Geometry: final body of the model. Coordinates: model frame, mm. A direction names the side the tool comes from. Give positions to 0.01 mm unless a question says otherwise; leave off trailing zeros. Write each loop counter-clockwise with the first axis right and the second up, starting at its lowest first coordinate (ties: lowest second). Pieces come first, ordered by that corner, then holes.
Q1. Reachability of faces 1 (the face through (2, 0, -5)), 2 (the face through (0, 25.4, 0)) from +Z, -Z, +X, -X, +Y, -Y: full face, straight path, thin tool, end or side. Return the list, or none.
Q2. Cut plane B-B on y = 4.5. Return the cut outline in (x, z), plus the area to 3 significant figures.
Q3. Cut plane C-C on x = 2.75. Return the cut outline in (y, z).
Q4. Pin query (flat end, axial travel): pin 1 (1.5 mm diameter, centred on y = 12, z = -2.5, fed in from +X); pin 2 (4 mm diameter, centred on x = -5, y = 16, fed in from +Z); pin 3 (4 mm diameter, centred on x = 1.5, y = 3.5, fed in from -Z); pin 4 (1.7 mm diameter, centred on x = -4.5, z = 5.5, fed in from -Y). Return the tip coordinate at first contact, or that it passes through.
Q5. Cut plane D-D on x = 4.25. Return the cut outline in (y, z), plus the area to 3 significant figures.
Q6. Cut plane A-A on x = 0. Return the cut outline in (y, z).
Q7. Line query: L1, parallel to X at y = 8.5, z = 0; L2, parallel to Z at x = 0.25, y = 1.25; L3, parallel to Y at x = -5, z = 2.25. Output: solid intervals per line, ascending.
```python
from build123d import *

# Parameters (mm, degrees)
SKETCH1_R           = 5.08
BOSS_EXTRUDE1_DEPTH = 25.4
BOSS_EXTRUDE2_DEPTH = 2
CUT_EXTRUDE1_DEPTH  = 0.1


with BuildPart() as part:
    # Sketch1 → Boss-Extrude1 (new body)
    with BuildSketch(Plane(origin=(0, 0, 0), x_dir=(1, 0, 0), z_dir=(0, 1, 0))):
        Circle(SKETCH1_R)
    extrude(amount=BOSS_EXTRUDE1_DEPTH)

    # Sketch2 → Boss-Extrude2 (add)
    with BuildSketch(Plane.XZ):
        Polygon((-7.332348419, 0), (-3.666174209, -6.35), (3.666174209, -6.35), (7.332348419, 0), (3.666174209, 6.35), (-3.666174209, 6.35), align=None)
    extrude(amount=BOSS_EXTRUDE2_DEPTH)

    # Sketch3 → Cut-Extrude1 (cut)
    with BuildSketch(Plane.XZ.offset(2)):
        Polygon((-4.979562137, 4.075145379), (-3.423879788, 6.35), (-3.666174209, 6.35), align=None)
        Polygon((0.86519926, 6.35), (3.786930674, 6.140843669), (3.666174209, 6.35), align=None)
        Polygon((6.052569822, 2.216641552), (7.211034583, -0.210121728), (7.332348419, 0), align=None)
        Polygon((4.91331885, -4.189882119), (3.423203754, -6.35), (3.666174209, -6.35), align=None)
        Polygon((-1.147445647, -6.35), (-3.787594099, -6.139694582), (-3.666174209, -6.35), align=None)
        Polygon((-6.07045658, -2.185660778), (-7.210941867, 0.210282315), (-7.332348419, 0), align=None)
    extrude(amount=-CUT_EXTRUDE1_DEPTH, mode=Mode.SUBTRACT)


solid = part.part
```
Data:
1. face 1: +Y
1. face 2: +Z, -Z, +X, -X, +Y
2. outline: circle Ø10.16 at (0, 0)
2. area: 81.1 mm2
3. outline: (-2, -6.35) - (0, -6.35) - (0, -4.27) - (25.4, -4.27) - (25.4, 4.27) - (0, 4.27) - (0, 6.35) - (-1.9, 6.35) - (-1.9, 6.22) - (-2, 6.22) - close
4. pin 1: stops at x = 4.77
4. pin 2: stops at z = 4.1
4. pin 3: stops at z = -5.08
4. pin 4: stops at y = -2
5. outline: (-2, -5.15) - (-1.9, -5.15) - (-1.9, -5.34) - (0, -5.34) - (0, -2.78) - (25.4, -2.78) - (25.4, 2.78) - (0, 2.78) - (0, 5.34) - (-2, 5.34) - close
5. area: 163 mm2
6. outline: (-2, -6.35) - (0, -6.35) - (0, -5.08) - (25.4, -5.08) - (25.4, 5.08) - (0, 5.08) - (0, 6.35) - (-2, 6.35) - close
7. L1: x = -5.08 to 5.08
7. L2: z = -5.07 to 5.07
7. L3: y = -2 to 0
